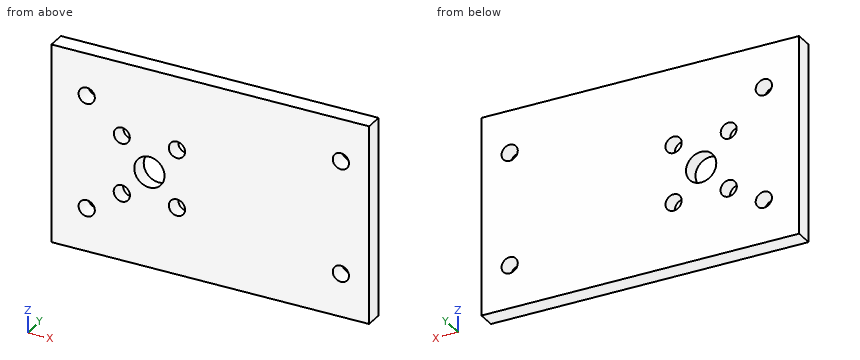
from build123d import *

# Parameters (mm, degrees)
SKETCH1_W           = 90
SKETCH1_H           = 56.23
BOSS_EXTRUDE1_DEPTH = 5
SKETCH2_R           = 2.3
CUT_EXTRUDE1_DEPTH  = 15
SKETCH7_R           = 2.3
CUT_EXTRUDE3_DEPTH  = 45
SKETCH12_R          = 2.257742522
SKETCH12_R_2        = 2.3
SKETCH12_R_3        = 4.287283452
CUT_EXTRUDE5_DEPTH  = 20


with BuildPart() as part:
    # Sketch1 → Boss-Extrude1 (new body)
    with BuildSketch(Plane(origin=(0, 0, 0), x_dir=(1, 0, 0), z_dir=(0, 1, 0))):
        with Locations((45, 28.115)):
            Rectangle(SKETCH1_W, SKETCH1_H)
    extrude(amount=BOSS_EXTRUDE1_DEPTH)

    # Sketch2 → Cut-Extrude1 (cut)
    with BuildSketch(Plane(origin=(0, 5, 0), x_dir=(1, 0, 0), z_dir=(0, 1, 0))):
        with Locations(Location((82, 12, 0), (0, 0, 270))):
            Circle(SKETCH2_R)
        with Locations(Location((10, 12, 0), (0, 0, 270))):
            Circle(SKETCH2_R)
    extrude(amount=-CUT_EXTRUDE1_DEPTH, mode=Mode.SUBTRACT)

    # Sketch7 → Cut-Extrude3 (cut)
    with BuildSketch(Plane(origin=(0, 5, 0), x_dir=(1, 0, 0), z_dir=(0, 1, 0))):
        with Locations(Location((82, 44, 0), (0, 0, 270))):
            Circle(SKETCH7_R)
        with Locations(Location((10, 44, 0), (0, 0, 270))):
            Circle(SKETCH7_R)
    extrude(amount=-CUT_EXTRUDE3_DEPTH, mode=Mode.SUBTRACT)

    # Sketch12 → Cut-Extrude5 (cut)
    with BuildSketch(Plane(origin=(0, 15.35002401, -2.983742412), x_dir=(-1, 0, 0), z_dir=(0, 0.9816271834476639, -0.19080899537654525))):
        with Locations(Location((-19.945482257, -20.397734662, 0), (0, 0, 270))):
            Circle(SKETCH12_R)
        with Locations(Location((-35.559756703, -20.397734662, 0), (0, 0, 270))):
            Circle(SKETCH12_R_2)
        with Locations(Location((-35.559756703, -36.512466621, 0), (0, 0, 270))):
            Circle(SKETCH12_R_2)
        with Locations(Location((-19.945482257, -36.512466621, 0), (0, 0, 270))):
            Circle(SKETCH12_R_2)
        with Locations(Location((-27.75261948, -28.605237896, 0), (0, 0, 270))):
            Circle(SKETCH12_R_3)
    extrude(amount=-CUT_EXTRUDE5_DEPTH, mode=Mode.SUBTRACT)


solid = part.part
Design review of the part built by this model. Coordinates are the model's own, in mm. Give positions to 0.01 mm unless a question says otherwise; leave off trailing zeros. Order: outer loops, then holes, each group sorted by start corner. A loop starts at its lowest first (then second) coordinate and runs counter-clockwise, first axis right, second up. Notation, with made-up numbers: (45.5, 52) - (89.5, 52) arc R19 ccw to (89.5, 61) - close; hole circle Ø7 at (49, 12.5). An arc over 180 degrees is marked (long way). Write item = value, one per line. Start each with the question number.
Q1. We need section A-A on z = -12. State the section outline as (x, y) points.
Q2. We need section C-C on y = 1.65. State how many separate pieces and enclosed holes the cut face has, plus the area to 3 significant figures.
Q3. We need section B-B on x = 82. State the section outline as (y, z) points, plus the area to 3 significant figures.
Q4. To check wall thickness, follow L1, parallel to X at y = 4.05, z = -44; L2, parallel to X at y = 0.5, z = -10.5; L3, parallel to X at y = 4.75, z = -31.5. State the ranges of each line that lie inside material, in increasing order. Write a range as from..to.
Working result:
q1.outline = (0, 0) - (7.7, 0) - (7.7, 5) - (0, 5) - close; (12.3, 0) - (79.7, 0) - (79.7, 5) - (12.3, 5) - close; (84.3, 0) - (90, 0) - (90, 5) - (84.3, 5) - close
q2.separate_pieces = 1
q2.enclosed_holes = 9
q2.area = 4,870 mm²
q3.outline = (0, -56.23) - (5, -56.23) - (5, -46.3) - (0, -46.3) - close; (0, -41.7) - (5, -41.7) - (5, -14.3) - (0, -14.3) - close; (0, -9.7) - (5, -9.7) - (5, 0) - (0, 0) - close
q3.area = 235 mm²
q4.L1 = 0..7.7, 12.3..79.7, 84.3..90
q4.L2 = 0..8.26, 11.74..80.26, 83.74..90
q4.L3 = 0..23.7, 31.8..90
